```python
from build123d import *

# Parameters (mm, degrees)
SKETCH_1_W       = 85
SKETCH_1_H       = 45
EXTRUDE_1_DEPTH  = 10
SKETCH_2_W       = 19
SKETCH_2_H       = 45
EXTRUDE_2_DEPTH  = 7.5
CHAMFER_1_SIZE   = 8
CHAMFER_1_SIZE_2 = 4.618802154
SKETCH_3_W       = 38.5
SKETCH_3_H       = 31.5
EXTRUDE_3_DEPTH  = 19
FILLET_1_R       = 2
CHAMFER_2_SIZE   = 1
FILLET_2_R       = 2


with BuildPart() as part:
    # 草图1 → 凸台-拉伸1 (new body)
    with BuildSketch(Plane(origin=(0, 0, 0), x_dir=(1, 0, 0), z_dir=(0, 1, 0))):
        Rectangle(SKETCH_1_W, SKETCH_1_H)
    extrude(amount=EXTRUDE_1_DEPTH)

    # 草图2 → 凸台-拉伸2 (add)
    with BuildSketch(Plane(origin=(0, 10, 0), x_dir=(1, 0, 0), z_dir=(0, 1, 0))):
        with Locations((-33, 0)):
            Rectangle(SKETCH_2_W, SKETCH_2_H)
    extrude(amount=EXTRUDE_2_DEPTH)

    # 倒角1
    # the kernel refuses this chamfer: 8, 4.618802154 mm, written as the material it adds along each edge
    with BuildSketch(Plane(origin=(-23.5, 10, -22.5), x_dir=(-0.01932676561270072, 0.9998132206222079, 0), z_dir=(0, 0, 1))) as chamfer_1_piece_1_section:
        Polygon((CHAMFER_1_SIZE * 0.999813220622, -CHAMFER_1_SIZE * 0.0193267656127), (-CHAMFER_1_SIZE_2 * 0.0193267656107, -CHAMFER_1_SIZE_2 * 0.999813220518), (0, 0), align=None)
    chamfer_1_piece_1 = extrude(amount=45, mode=Mode.PRIVATE)
    chamfer_1_piece_1 = split(chamfer_1_piece_1, bisect_by=Plane(origin=(-21.997429692, 17.5, 0), z_dir=(0, -1, 0)), keep=Keep.TOP, mode=Mode.PRIVATE)
    add(chamfer_1_piece_1)

    # 草图3 → 凸台-拉伸3 (add)
    with BuildSketch(Plane(origin=(0, 10, 0), x_dir=(1, 0, 0), z_dir=(0, 1, 0))):
        with Locations((5.25, 0)):
            Rectangle(SKETCH_3_W, SKETCH_3_H)
    extrude(amount=EXTRUDE_3_DEPTH)

    # 圆角1
    fillet_1_edges = [part.edges().sort_by_distance(p)[0] for p in [
        (-14, 19.5, -15.75),
        (-14, 19.5, 15.75),
        (24.5, 19.5, 15.75),
        (24.5, 19.5, -15.75),
    ]]
    fillet(fillet_1_edges, radius=FILLET_1_R)

    # 倒角2
    chamfer_2_edges = [part.edges().sort_by_distance(p)[0] for p in [
        (-14, 29, 0),
        (5.25, 29, -15.75),
        (5.25, 29, 15.75),
        (24.5, 29, 0),
        (-13.414213562, 29, 15.164213562),
        (23.914213562, 29, 15.164213562),
        (23.914213562, 29, -15.164213562),
        (-13.414213562, 29, -15.164213562),
    ]]
    chamfer(chamfer_2_edges, length=CHAMFER_2_SIZE)

    # 圆角2
    fillet_2_edges = [part.edges().sort_by_distance(p)[0] for p in [
        (-42.5, 8.75, -22.5),
        (42.5, 5, -22.5),
        (42.5, 5, 22.5),
        (-42.5, 8.75, 22.5),
    ]]
    fillet(fillet_2_edges, radius=FILLET_2_R)


solid = part.part
```
The listing builds one solid part. Answer for the finished solid, in the listing's coordinates (mm). A direction names the side the tool comes from. Give positions to 0.01 mm unless a question says otherwise; leave off trailing zeros. Write each loop counter-clockwise with the first axis right and the second up, starting at its lowest first coordinate (ties: lowest second). Pieces come first, ordered by that corner, then holes. Notation, with made-up numbers: (44.25, 47.5) -> (102.25, 47.5) arc R17 cw to (102.25, 57.5) -> close; hole circle Ø7 at (48.5, 61). An arc over 180 degrees is marked (long way). Write item = value, one per line. Start each with the question number.
1) Straight lines are drawn through the part: line 1 along Y through (x, z) = (-33, 4); line 2 along Y through (x, z) = (32, -8); line 3 along Z through (x, y) = (3, 21.5). For each, find the intervals that lie inside material, in ascending order.
2) Determine the mould class of faces 6 (the face through (-13.4, 19.13, -15.18)), 7 (the face through (-1, 7, 22.5)), 8 (the face through (-21.077, 13.802, -0.315)), 9 (the face through (-42.5, 9, 0)) for opening direction X: +X half, -X half, draft (parallel to the pull), parting line (faces both ways), or undercut.
3) The part is cut by section C-C, the plane z = -5. Determine the outline of the cut face in (x, y), and give its area (3 significant figures).
4) The part is cut by section A-A, the plane y = 25.25. Determine the outline of the cut face in (x, z), and give its area (3 significant figures).
5) Each of these flat-tipped pins is pushed along its axis until it touches: pin 1 (1.5 mm diameter, centred on y = 19.5, z = 12, fed in from +X); pin 2 (9.5 mm diameter, centred on x = -33, z = -9.5, fed in from +Y); pin 3 (5.5 mm diameter, centred on x = 9.5, y = 22.5, fed in from +Z). Where does it stop, or does it pass through?
6) The part is cut by section D-D, the plane x = 2.5. Determine the outline of the cut face in (y, z).
7) The part is cut by section B-B, the plane y = 14.5. Determine the outline of the cut face in (x, z), and give its area (3 significant figures).
8) Which of the six approach directions +Z, -Z, +X, -X, +Y, -Y give full straight-line access (tool end or side, diameter ignored) to faces 1 (the face through (23.9, 19.13, 15.18)), 2 (the face through (-33, 17.5, 0)), 3 (the face through (-13.4, 19.13, 15.18)), 4 (the face through (24.5, 19, 0)), 5 (the face through (5, 19, -15.75))?
Solutions:
q1.line_1 = 0 to 17.5
q1.line_2 = 0 to 10
q1.line_3 = -15.75 to 15.75
q2.face_6 = undercut
q2.face_7 = draft
q2.face_8 = undercut
q2.face_9 = -X half
q3.outline = (-42.5, 0) -> (42.5, 0) -> (42.5, 10) -> (24.5, 10) -> (24.5, 28) -> (23.5, 29) -> (-13, 29) -> (-14, 28) -> (-14, 10) -> (-18.88, 10) -> (-23.21, 17.5) -> (-42.5, 17.5) -> close
q3.area = 1,740 mm²
q4.outline = (-14, -13.75) arc R2 ccw to (-12, -15.75) -> (22.5, -15.75) arc R2 ccw to (24.5, -13.75) -> (24.5, 13.75) arc R2 ccw to (22.5, 15.75) -> (-12, 15.75) arc R2 ccw to (-14, 13.75) -> close
q4.area = 1,210 mm²
q5.pin_1 = 24.5
q5.pin_2 = 17.5
q5.pin_3 = 15.75
q6.outline = (0, -22.5) -> (10, -22.5) -> (10, -15.75) -> (28, -15.75) -> (29, -14.75) -> (29, 14.75) -> (28, 15.75) -> (10, 15.75) -> (10, 22.5) -> (0, 22.5) -> close
q7.outline = (-42.5, -20.5) arc R2 ccw to (-40.5, -22.5) -> (-21.48, -22.5) -> (-21.48, 22.5) -> (-40.5, 22.5) arc R2 ccw to (-42.5, 20.5) -> close; (-14, -13.75) arc R2 ccw to (-12, -15.75) -> (22.5, -15.75) arc R2 ccw to (24.5, -13.75) -> (24.5, 13.75) arc R2 ccw to (22.5, 15.75) -> (-12, 15.75) arc R2 ccw to (-14, 13.75) -> close
q7.area = 2,150 mm²
q8.face_1 = +Z, +X, +Y
q8.face_2 = +Z, -Z, -X, +Y
q8.face_3 = +Z, +Y
q8.face_4 = +Z, -Z, +X, +Y
q8.face_5 = -Z, +X, +Y
